Verification items for the finished model (mm, model axes). A direction names the side the tool comes from. Round coordinates to 2 decimals unless told otherwise and drop trailing zeros. Loops run counter-clockwise (first coordinate to the right, second up) from the corner with the lowest first, then second, coordinate; pieces in that order, holes last. Notation, with made-up numbers: (36.25, 24) -> (48.25, 24) arc R25 ccw to (48.25, 47) -> close; hole circle Ø7 at (-0.5, 49). An arc over 180 degrees is marked (long way). Use a Markdown table: item, result. Add a question column.
```python
from build123d import *

# Parameters (mm, degrees)
SKETCH_1_W          = 14
SKETCH_1_H          = 4
SKETCH_1_W_2        = 98
SKETCH_1_H_2        = 68
EXTRUDE_1_DEPTH     = 4
SKETCH_2_R          = 1.5
CUT_EXTRUDE_1_DEPTH = 4
SKETCH_3_R          = 1.5
SKETCH_3_W          = 4.2
SKETCH_3_H          = 12
CUT_EXTRUDE_2_DEPTH = 10
CUT_EXTRUDE_3_DEPTH = 5
FILLET_1_R          = 3


with BuildPart() as part:
    # 草图1 → 凸台-拉伸1 (new body)
    with BuildSketch(Plane(origin=(0, 0, 0), x_dir=(1, 0, 0), z_dir=(0, 1, 0))):
        with Locations((-35, -36)):
            Rectangle(SKETCH_1_W, SKETCH_1_H)
        Rectangle(SKETCH_1_W_2, SKETCH_1_H_2)
        with Locations((0, -36)):
            Rectangle(SKETCH_1_W, SKETCH_1_H)
        with Locations((35, -36)):
            Rectangle(SKETCH_1_W, SKETCH_1_H)
        with Locations((-35, 36)):
            Rectangle(SKETCH_1_W, SKETCH_1_H)
        with Locations((35, 36)):
            Rectangle(SKETCH_1_W, SKETCH_1_H)
        with Locations((0, 36)):
            Rectangle(SKETCH_1_W, SKETCH_1_H)
    extrude(amount=EXTRUDE_1_DEPTH)

    # 草图2 → 切除-拉伸1 (cut)
    with BuildSketch(Plane(origin=(0, 4, 0), x_dir=(1, 0, 0), z_dir=(0, 1, 0))):
        with Locations((-43.5, 34)):
            Circle(SKETCH_2_R)
        with Locations((-26.5, 34)):
            Circle(SKETCH_2_R)
        with Locations((-8.5, 34)):
            Circle(SKETCH_2_R)
        with Locations((-43.5, -34)):
            Circle(SKETCH_2_R)
        with Locations((-26.5, -34)):
            Circle(SKETCH_2_R)
        with Locations((-8.5, -34)):
            Circle(SKETCH_2_R)
        with Locations((8.5, 34)):
            Circle(SKETCH_2_R)
        with Locations((26.5, 34)):
            Circle(SKETCH_2_R)
        with Locations((26.5, -34)):
            Circle(SKETCH_2_R)
        with Locations((8.5, -34)):
            Circle(SKETCH_2_R)
        with Locations((43.5, -34)):
            Circle(SKETCH_2_R)
        with Locations((43.5, 34)):
            Circle(SKETCH_2_R)
    extrude(amount=-CUT_EXTRUDE_1_DEPTH, mode=Mode.SUBTRACT)

    # 草图3 → 切除-拉伸2 (cut)
    with BuildSketch(Plane(origin=(0, 4, 0), x_dir=(1, 0, 0), z_dir=(0, 1, 0))):
        with Locations((45.1, 10.5)):
            Circle(SKETCH_3_R)
        with Locations((45.1, 19.5)):
            Circle(SKETCH_3_R)
        with Locations((40.9, 19.5)):
            Circle(SKETCH_3_R)
        with Locations((40.9, 10.5)):
            Circle(SKETCH_3_R)
        with Locations((43, 15)):
            Rectangle(SKETCH_3_W, SKETCH_3_H)
        with BuildLine():
            ThreePointArc((42.4, 10.5), (41.960660172, 11.560660172), (40.9, 12))
            Line((40.9, 12), (40.9, 9))
            ThreePointArc((40.9, 9), (41.960660172, 9.439339828), (42.4, 10.5))
        make_face()
        with BuildLine():
            Line((40.9, 9), (40.9, 12))
            ThreePointArc((40.9, 12), (39.4, 10.5), (40.9, 9))
        make_face()
        with BuildLine():
            ThreePointArc((42.4, 19.5), (41.960660172, 20.560660172), (40.9, 21))
            Line((40.9, 21), (40.9, 18))
            ThreePointArc((40.9, 18), (41.960660172, 18.439339828), (42.4, 19.5))
        make_face()
        with BuildLine():
            Line((40.9, 18), (40.9, 21))
            ThreePointArc((40.9, 21), (39.4, 19.5), (40.9, 18))
        make_face()
        with BuildLine():
            ThreePointArc((46.6, 19.5), (46.160660172, 20.560660172), (45.1, 21))
            Line((45.1, 21), (45.1, 18))
            ThreePointArc((45.1, 18), (46.160660172, 18.439339828), (46.6, 19.5))
        make_face()
        with BuildLine():
            Line((45.1, 18), (45.1, 21))
            ThreePointArc((45.1, 21), (43.6, 19.5), (45.1, 18))
        make_face()
        with BuildLine():
            ThreePointArc((46.6, 10.5), (46.160660172, 11.560660172), (45.1, 12))
            Line((45.1, 12), (45.1, 9))
            ThreePointArc((45.1, 9), (46.160660172, 9.439339828), (46.6, 10.5))
        make_face()
        with BuildLine():
            Line((45.1, 9), (45.1, 12))
            ThreePointArc((45.1, 12), (43.6, 10.5), (45.1, 9))
        make_face()
        with BuildLine():
            ThreePointArc((40.9, -18), (39.4, -19.5), (40.9, -21))
            Line((40.9, -21), (40.9, -18))
        make_face()
        with BuildLine():
            Line((40.9, -18), (40.9, -21))
            ThreePointArc((40.9, -21), (41.960660172, -20.560660172), (42.4, -19.5))
            ThreePointArc((42.4, -19.5), (41.960660172, -18.439339828), (40.9, -18))
        make_face()
        with Locations((40.9, -19.5)):
            Circle(SKETCH_3_R)
        with Locations((45.1, -19.5)):
            Circle(SKETCH_3_R)
        with Locations((45.1, -10.5)):
            Circle(SKETCH_3_R)
        with Locations((40.9, -10.5)):
            Circle(SKETCH_3_R)
        with Locations((43, -15)):
            Rectangle(SKETCH_3_W, SKETCH_3_H)
        with BuildLine():
            ThreePointArc((45.1, -18), (43.6, -19.5), (45.1, -21))
            Line((45.1, -21), (45.1, -18))
        make_face()
        with BuildLine():
            Line((45.1, -18), (45.1, -21))
            ThreePointArc((45.1, -21), (46.160660172, -20.560660172), (46.6, -19.5))
            ThreePointArc((46.6, -19.5), (46.160660172, -18.439339828), (45.1, -18))
        make_face()
        with BuildLine():
            ThreePointArc((40.9, -9), (39.4, -10.5), (40.9, -12))
            Line((40.9, -12), (40.9, -9))
        make_face()
        with BuildLine():
            Line((40.9, -9), (40.9, -12))
            ThreePointArc((40.9, -12), (41.960660172, -11.560660172), (42.4, -10.5))
            ThreePointArc((42.4, -10.5), (41.960660172, -9.439339828), (40.9, -9))
        make_face()
        with BuildLine():
            ThreePointArc((45.1, -9), (43.6, -10.5), (45.1, -12))
            Line((45.1, -12), (45.1, -9))
        make_face()
        with BuildLine():
            Line((45.1, -9), (45.1, -12))
            ThreePointArc((45.1, -12), (46.160660172, -11.560660172), (46.6, -10.5))
            ThreePointArc((46.6, -10.5), (46.160660172, -9.439339828), (45.1, -9))
        make_face()
    cut_extrude_2 = extrude(amount=-CUT_EXTRUDE_2_DEPTH, mode=Mode.SUBTRACT)

    # 镜向1: 切除-拉伸2 across plane
    add(cut_extrude_2.mirror(Plane(origin=(0, 0, 0), x_dir=(0, 0, 1), z_dir=(1, 0, 0))), mode=Mode.SUBTRACT)

    # 草图4 → 切除-拉伸3 (cut)
    with BuildSketch(Plane(origin=(0, 4, 0), x_dir=(1, 0, 0), z_dir=(0, 1, 0))):
        Polygon((-24.454122256, 0), (-38, 19.048890577), (-38, -19.048890577), align=None)
        Polygon((-8.454122256, 22.5), (-35.545877744, 22.5), (-22, 3.451109423), align=None)
        Polygon((-6, 19.048890577), (-19.545877744, 0), (-6, -19.048890577), align=None)
        Polygon((-8.454122256, -22.5), (-22, -3.451109423), (-35.545877744, -22.5), align=None)
        Polygon((19.545877744, 0), (6, 19.048890577), (6, -19.048890577), align=None)
        Polygon((8.454122256, 22.5), (22, 3.451109423), (35.545877744, 22.5), align=None)
        Polygon((38, 19.048890577), (24.454122256, 0), (38, -19.048890577), align=None)
        Polygon((35.545877744, -22.5), (22, -3.451109423), (8.454122256, -22.5), align=None)
    extrude(amount=-CUT_EXTRUDE_3_DEPTH, mode=Mode.SUBTRACT)

    # 圆角1
    fillet_1_edges = [part.edges().sort_by_distance(p)[0] for p in [
        (6, 2, -19.048890577),
        (19.545877744, 2, 0),
        (6, 2, 19.048890577),
        (-22, 2, 3.451109423),
        (-8.454122256, 2, 22.5),
        (-35.545877744, 2, 22.5),
        (-8.454122256, 2, -22.5),
        (-22, 2, -3.451109423),
        (-35.545877744, 2, -22.5),
        (-6, 2, -19.048890577),
        (-6, 2, 19.048890577),
        (-19.545877744, 2, 0),
        (35.545877744, 2, 22.5),
        (8.454122256, 2, 22.5),
        (22, 2, 3.451109423),
        (35.545877744, 2, -22.5),
        (22, 2, -3.451109423),
        (8.454122256, 2, -22.5),
        (38, 2, -19.048890577),
        (38, 2, 19.048890577),
        (24.454122256, 2, 0),
        (-24.454122256, 2, 0),
        (-38, 2, 19.048890577),
        (-38, 2, -19.048890577),
    ]]
    fillet(fillet_1_edges, radius=FILLET_1_R)


solid = part.part
```
1) Sectioned sample at C-C on z = -15. Enter the section's corners in (x, y).
2) Access from +Z, -Z, +X, -X, +Y, -Y to the whole of each face (thin tool, end or side, straight path). Record for faces 1 (the face through (-7, 2, -36)), 2 (the face through (49, 2, 0)), 3 (the face through (40.9, 2, 15)).
3) Thickness scan on line 1 (X direction, y = 3.8, z = 1); line 2 (X direction, y = 2.6, z = 4.5); line 3 (X direction, y = 0.8, z = 22). Record the ranges inside material, lowest first.
4) Release check for a two-part mould opening along Z. For faces 4 (the face through (0, 2, 38)), 5 (the face through (42, 2, -36)), 6 (the face through (35, 2, -38)), 7 (the face through (43, 2, -9)) record: released by +Z, released by -Z, zero draft, split by the parting line, or undercut.
5) Sectioned sample at D-D on y = 0.7. State how many separate pieces and enclosed holes the cut face has, then the cut area to 3 significant figures.
6) Sectioned sample at B-B on x = -9. Enter the section's corners in (y, z), then the cut area to 3 significant figures.
7) Go/stop test with flat-tipped pins: pin 1 (2 mm diameter, centred on x = 19.5, y = 1, fed in from +Z); pin 2 (2 mm diameter, centred on y = 2.5, z = 36.5, fed in from +X); pin 3 (2 mm diameter, centred on x = -19, y = 2.5, fed in from -Z). Record where each tip stops, or that it passes through.
8) Sectioned sample at A-A on x = 43.5. Enter the section's corners in (y, z).
Geometry results:
| question | item | result |
|---|---|---|
| 1 | outline | (-49, 0) -> (-45.1, 0) -> (-45.1, 4) -> (-49, 4) -> close; (-40.9, 0) -> (-30.21, 0) -> (-30.21, 4) -> (-40.9, 4) -> close; (-13.79, 0) -> (13.79, 0) -> (13.79, 4) -> (-13.79, 4) -> close; (30.21, 0) -> (40.9, 0) -> (40.9, 4) -> (30.21, 4) -> close; (45.1, 0) -> (49, 0) -> (49, 4) -> (45.1, 4) -> close |
| 2 | face 1 | -Z, +Y, -Y |
| 2 | face 2 | +Z, -Z, +X, +Y, -Y |
| 2 | face 3 | +Y, -Y |
| 3 | line 1 | -49 to -38, -25.31 to -18.69, -6 to 6, 18.69 to 25.31, 38 to 49 |
| 3 | line 2 | -49 to -38, -27.65 to -16.35, -6 to 6, 16.35 to 27.65, 38 to 49 |
| 3 | line 3 | -49 to -31.39, -12.61 to 12.61, 31.39 to 49 |
| 4 | face 4 | released by +Z |
| 4 | face 5 | zero draft |
| 4 | face 6 | released by -Z |
| 4 | face 7 | undercut |
| 5 | separate pieces | 1 |
| 5 | enclosed holes | 12 |
| 5 | area | 4,850 mm^2 |
| 6 | outline | (0, -32.59) -> (4, -32.59) -> (4, -12.65) -> (0, -12.65) -> close; (0, 12.65) -> (4, 12.65) -> (4, 32.59) -> (0, 32.59) -> close |
| 6 | area | 159 mm^2 |
| 7 | pin 1 | z = 34 |
| 7 | pin 2 | x = 42 |
| 7 | pin 3 | z = -34 |
| 8 | outline | (0, -32.5) -> (4, -32.5) -> (4, -21) -> (0, -21) -> close; (0, -9) -> (4, -9) -> (4, 9) -> (0, 9) -> close; (0, 21) -> (4, 21) -> (4, 32.5) -> (0, 32.5) -> close |
